```python
from build123d import *

# Parameters (mm, degrees)
ESQUISSE1_W             = 49.5
ESQUISSE1_H             = 51.2
BOSS_EXTRU_1_DEPTH      = 1
ESQUISSE2_W             = 11.3
ESQUISSE2_H             = 6
ESQUISSE2_W_2           = 19.8
ESQUISSE2_H_2           = 17.2
ENL_V_MAT_EXTRU_1_DEPTH = 5
ESQUISSE4_W             = 5
ESQUISSE4_H             = 5
BOSS_EXTRU_3_DEPTH      = 16
ESQUISSE5_W             = 2.5
ESQUISSE5_H             = 5
BOSS_EXTRU_4_DEPTH      = 16
ESQUISSE6_W             = 5
ESQUISSE6_H             = 5
BOSS_EXTRU_5_DEPTH      = 16
ESQUISSE7_W             = 4
ESQUISSE7_H             = 4
BOSS_EXTRU_6_DEPTH      = 16


with BuildPart() as part:
    # Esquisse1 → Boss.-Extru.1 (new body)
    with BuildSketch(Plane.XY):
        with Locations((-1.366863252, -9.011290323)):
            Rectangle(ESQUISSE1_W, ESQUISSE1_H)
    extrude(amount=BOSS_EXTRU_1_DEPTH)

    # Esquisse2 → Enlèv. mat.-Extru.1 (cut)
    with BuildSketch(Plane.XY.offset(1)):
        with Locations((11.733136748, -31.611290323)):
            Rectangle(ESQUISSE2_W, ESQUISSE2_H)
        with Locations((-1.316863252, 7.988709677)):
            Rectangle(ESQUISSE2_W_2, ESQUISSE2_H_2)
    extrude(amount=-ENL_V_MAT_EXTRU_1_DEPTH, mode=Mode.SUBTRACT)

    # Esquisse4 → Boss.-Extru.3 (add)
    with BuildSketch(Plane(origin=(0, 0, 0), x_dir=(-1, 0, 0), z_dir=(0, 0, -1))):
        with Locations((20.616863252, 11.088709677)):
            Rectangle(ESQUISSE4_W, ESQUISSE4_H)
    extrude(amount=BOSS_EXTRU_3_DEPTH)

    # Esquisse5 → Boss.-Extru.4 (add)
    with BuildSketch(Plane(origin=(0, 0, 0), x_dir=(-1, 0, 0), z_dir=(0, 0, -1))):
        with Locations((-18.633136748, -30.111290323)):
            Rectangle(ESQUISSE5_W, ESQUISSE5_H)
    extrude(amount=BOSS_EXTRU_4_DEPTH)

    # Esquisse6 → Boss.-Extru.5 (add)
    with BuildSketch(Plane(origin=(0, 0, 0), x_dir=(-1, 0, 0), z_dir=(0, 0, -1))):
        with Locations((-17.883136748, 11.088709677)):
            Rectangle(ESQUISSE6_W, ESQUISSE6_H)
    extrude(amount=BOSS_EXTRU_5_DEPTH)

    # Esquisse7 → Boss.-Extru.6 (add)
    with BuildSketch(Plane(origin=(0, 0, 0), x_dir=(-1, 0, 0), z_dir=(0, 0, -1))):
        with Locations((21.116863252, -29.611290323)):
            Rectangle(ESQUISSE7_W, ESQUISSE7_H)
    extrude(amount=BOSS_EXTRU_6_DEPTH)


solid = part.part
```
Work out the finished part from the listing and answer in its coordinate system (mm). A direction names the side the tool comes from. Give positions to 0.01 mm unless a question says otherwise; leave off trailing zeros. Write each loop counter-clockwise with the first axis right and the second up, starting at its lowest first coordinate (ties: lowest second). Pieces come first, ordered by that corner, then holes.
(1) Flat-ended cylindrical pins translate along their axes: pin 1 Ø2.5 at (y, z) = (10.5, -6.5) entering from -X; pin 2 Ø1.5 at (x, y) = (-5.5, 0.5) entering from +Z; pin 3 Ø5.5 at (x, z) = (-20.5, -10.5) entering from +Y; pin 4 Ø4.5 at (y, z) = (-30.5, -10.5) entering from +X. Find the tip coordinate at first contact, or state that the pin passes through.
Final values:
pin 1: stops at x = -23.12
pin 2: passes through
pin 3: stops at y = 13.59
pin 4: stops at x = 19.88
(2) The part is cut by section D-D on y = -18.5. Write down the section's boundary in (x, z), plus the area to 3 significant figures.
Final values:
outline: (-26.12, 0) - (23.38, 0) - (23.38, 1) - (-26.12, 1) - close
area: 49.5 mm2
(3) Straight lines are drawn through the part: line 1 (Y direction, x = 19, z = -1.5); line 2 (X direction, y = 12, z = -11); line 3 (X direction, y = -30.5, z = -13). For each, find the intervals that lie inside material, in ascending order.
Final values:
line 1: y = -32.61 to -27.61, 8.59 to 13.59
line 2: x = -23.12 to -18.12, 15.38 to 20.38
line 3: x = -23.12 to -19.12, 17.38 to 19.88
(4) The part is cut by section C-C on x = -12. Write down the section's boundary in (y, z), plus the area to 3 significant figures.
Final values:
outline: (-34.61, 0) - (16.59, 0) - (16.59, 1) - (-34.61, 1) - close
area: 51.2 mm2
(5) Which of the six approach directions +Z, -Z, +X, -X, +Y, -Y give full straight-line access (tool end or side, diameter ignored) to faces 1 (the flat face through (19.883, -30, -8)), 2 (the flat face through (18, 8.589, -8)), 3 (the flat face through (-19.117, -30, -8))?
Final values:
face 1: -Z, +X, -Y
face 2: -Z, +X, -X
face 3: -Z, -Y
(6) The part is cut by section A-A on y = 8. Write down the section's boundary in (x, z), plus the area to 3 significant figures.
Final values:
outline: (-26.12, 0) - (-11.22, 0) - (-11.22, 1) - (-26.12, 1) - close; (8.58, 0) - (23.38, 0) - (23.38, 1) - (8.58, 1) - close
area: 29.7 mm2
(7) The part is cut by section B-B on z = -11. Write down the section's boundary in (x, y).
Final values:
outline: (-23.12, -31.61) - (-19.12, -31.61) - (-19.12, -27.61) - (-23.12, -27.61) - close; (-23.12, 8.59) - (-18.12, 8.59) - (-18.12, 13.59) - (-23.12, 13.59) - close; (15.38, 8.59) - (20.38, 8.59) - (20.38, 13.59) - (15.38, 13.59) - close; (17.38, -32.61) - (19.88, -32.61) - (19.88, -27.61) - (17.38, -27.61) - close
(8) The mould has two halves that part along Y. Classify faces 4 (the flat face through (19, -27.611, -8)), 5 (the flat face through (18, 13.589, -8)), 6 (the flat face through (15.383, 11, -8)): pulls with the +Y half, pulls with the -Y half, needs draft (parallel to the pull), parting line crosses it, or undercut.
Final values:
face 4: undercut
face 5: pulls with the +Y half
face 6: needs draft
